from build123d import *

# Parameters (mm, degrees)
SKETCH1_R               = 6.5
SKETCH1_R_2             = 5
BOSS_EXTRUDE1_DEPTH     = 25
BOSS_EXTRUDE2_DEPTH     = 2
CUT_EXTRUDE1_DEPTH      = 29.075790283
CUT_EXTRUDE1_DEPTH_BACK = 29.075790283
SKETCH4_R               = 2
SKETCH3_W               = 28
SKETCH3_H               = 13
SKETCH3_R               = 3
BOSS_EXTRUDE3_DEPTH     = 8.5
SKETCH5_R               = 5
CUT_EXTRUDE2_DEPTH      = 5
CHAMFER1_SIZE2          = 4
CHAMFER1_SIZE           = 9


with BuildPart() as part:
    # Sketch1 → Boss-Extrude1 (new body)
    with BuildSketch(Plane(origin=(0, 0, 0), x_dir=(0, 0, -1), z_dir=(1, 0, 0))):
        Circle(SKETCH1_R)
        Circle(SKETCH1_R_2, mode=Mode.SUBTRACT)
    extrude(amount=BOSS_EXTRUDE1_DEPTH)

    # Sketch2 → Boss-Extrude2 (add)
    with BuildSketch(Plane(origin=(0, 0, 0), x_dir=(0, 0, -1), z_dir=(1, 0, 0))):
        Polygon((-6.5, -6.5), (-6.5, -11), (6.5, -11), (6.5, -6.5), (6.5, 6.5), (-6.5, 6.5), align=None)
    extrude(amount=-BOSS_EXTRUDE2_DEPTH)

    # Sketch4 → Cut-Extrude1 (cut, two sides: drawn at the far end of the back side and taken through both)
    with BuildSketch(Plane(origin=(0, 0, 0), x_dir=(1, 0, 0), z_dir=(0, 1, 0)).offset(-CUT_EXTRUDE1_DEPTH_BACK)):
        with Locations(Location((10, 0, 0), (0, 0, 270))):
            Circle(SKETCH4_R)
        with Locations(Location((20, 0, 0), (0, 0, 270))):
            Circle(SKETCH4_R)
    extrude(amount=CUT_EXTRUDE1_DEPTH + CUT_EXTRUDE1_DEPTH_BACK, mode=Mode.SUBTRACT)

    # Sketch3 → Boss-Extrude3 (add)
    with BuildSketch(Plane(origin=(0, -2.5, 0), x_dir=(1, 0, 0), z_dir=(0, 1, 0))):
        with Locations((-16, 0)):
            Rectangle(SKETCH3_W, SKETCH3_H)
        with Locations(Location((-17, 0, 0), (0, 0, 270))):
            Circle(SKETCH3_R, mode=Mode.SUBTRACT)
    extrude(amount=-BOSS_EXTRUDE3_DEPTH)

    # Sketch5 → Cut-Extrude2 (cut)
    with BuildSketch(Plane.XZ.offset(11)):
        with Locations(Location((-17, 0, 0), (0, 0, 270))):
            Circle(SKETCH5_R)
    extrude(amount=-CUT_EXTRUDE2_DEPTH, mode=Mode.SUBTRACT)

    # Chamfer1
    chamfer1_edges = [part.edges().sort_by_distance(p)[0] for p in [
        (-2, -2.5, 0),
    ]]
    chamfer1_side = [part.faces().sort_by_distance(p)[0] for p in [
        (-2, -2.42, 0),
    ]]
    chamfer(chamfer1_edges, length=CHAMFER1_SIZE - 0.0001, length2=CHAMFER1_SIZE2 - 0.0001, reference=chamfer1_side[0])  # a hair under: the kernel refuses the full size


solid = part.part
Read the model definition and answer for the solid it produces. Units are mm, in the model's axes. A direction names the side the tool comes from. Coordinates: 2 decimals unless noted, no trailing zeros. Order: outer loops, then holes, each group sorted by start corner. A loop starts at its lowest first (then second) coordinate and runs counter-clockwise, first axis right, second up. Notation, with made-up numbers: (6.25, -16.5) -> (24.25, -16.5) arc R25 ccw to (24.25, -2.5) -> close; hole circle Ø10 at (79, 36.5). An arc over 180 degrees is marked (long way). Answer as a JSON object with one key per item and string values.
1) A cutting plane is placed at B-B, the plane y = -3.5. Determine the outline of the cut face in (x, z), plus the area to 3 significant figures.
Model answer:
{"outline": "(-30, -6.5) -> (0, -6.5) -> (0, -5.48) -> (25, -5.48) -> (25, -3.57) -> (0, -3.57) -> (0, 3.57) -> (25, 3.57) -> (25, 5.48) -> (0, 5.48) -> (0, 6.5) -> (-30, 6.5) -> close; hole circle Ø6 at (-17, 0)", "area": "457 mm²"}
2) A tool of negligible diameter and unlimited length cuts with its end or side. For faces 1 (the face through (12.32, 1.95, -6.2)), 2 (the face through (0, 5, -5)), 3 (the face through (-21.88, -8.54, 1.08)), from which of +Z, -Z, +X, -X, +Y, -Y can it reach the whole face along a straight path? Write none if from no direction.
Model answer:
{"face 1": "+X", "face 2": "-Z, +X, +Y", "face 3": "-Y"}
3) The mould has two halves that part along X. Classify faces 4 (the face through (9.234, -5.559, 1.847)), 5 (the face through (-4, 2, 0)), 6 (the face through (0, -8, 0)): released by +X, released by -X, zero draft, split by the parting line, or undercut.
Model answer:
{"face 4": "undercut", "face 5": "released by -X", "face 6": "released by +X"}
4) Each of these flat-tipped pins is pushed along its axis until it touches: pin 1 (5 mm diameter, centred on x = -17.5, z = 1.5, fed in from -Y); pin 2 (3 mm diameter, centred on y = -0.5, z = 1.5, fed in from -X); pin 3 (4 mm diameter, centred on x = 4.5, y = -4.5, fed in from -Z). Where does it stop, or does it pass through?
Model answer:
{"pin 1": "stops at y = -6", "pin 2": "stops at x = -5.78", "pin 3": "stops at z = -6"}
5) A cutting plane is placed at C-C, the plane x = 3.5. Determine the outline of the cut face in (y, z).
Model answer:
{"outline": "circle Ø13 at (0, 0); hole circle Ø10 at (0, 0)"}
6) Consider line 1 along Z through (x, y) = (-15, -8.5); line 2 along X through (y, z) = (-5.9, 0); line 3 along Z through (x, y) = (17, 0.25). Determine where each line is inside the solid, lowest interval first. Write a range as from..to.
Model answer:
{"line 1": "z = -6.5..-4.58, 4.58..6.5", "line 2": "x = -30..-20, -14..8, 12..18, 22..25", "line 3": "z = -6.5..-4.99, 4.99..6.5"}
7) A cutting plane is placed at A-A, the plane x = -17. Determine the outline of the cut face in (y, z).
Model answer:
{"outline": "(-11, -6.5) -> (-2.5, -6.5) -> (-2.5, -3) -> (-6, -3) -> (-6, -5) -> (-11, -5) -> close; (-11, 5) -> (-6, 5) -> (-6, 3) -> (-2.5, 3) -> (-2.5, 6.5) -> (-11, 6.5) -> close"}
